Study the drawing (mm; zero at the part's minimum x, y, z) and answer. A direction names the side the tool comes from. Round coordinates to 2 decimals unless told otherwise and drop trailing zeros. Order: outer loops, then holes, each group sorted by start corner. A loop starts at its lowest first (then second) coordinate and runs counter-clockwise, first axis right, second up. Notation, with made-up numbers: (84, 76.25) - (97, 76.25) arc R27 ccw to (97, 110.25) - close; hole circle Ø1 at (-24, 48.5). An arc over 180 degrees is marked (long way). Put each result on its own line as item: value.
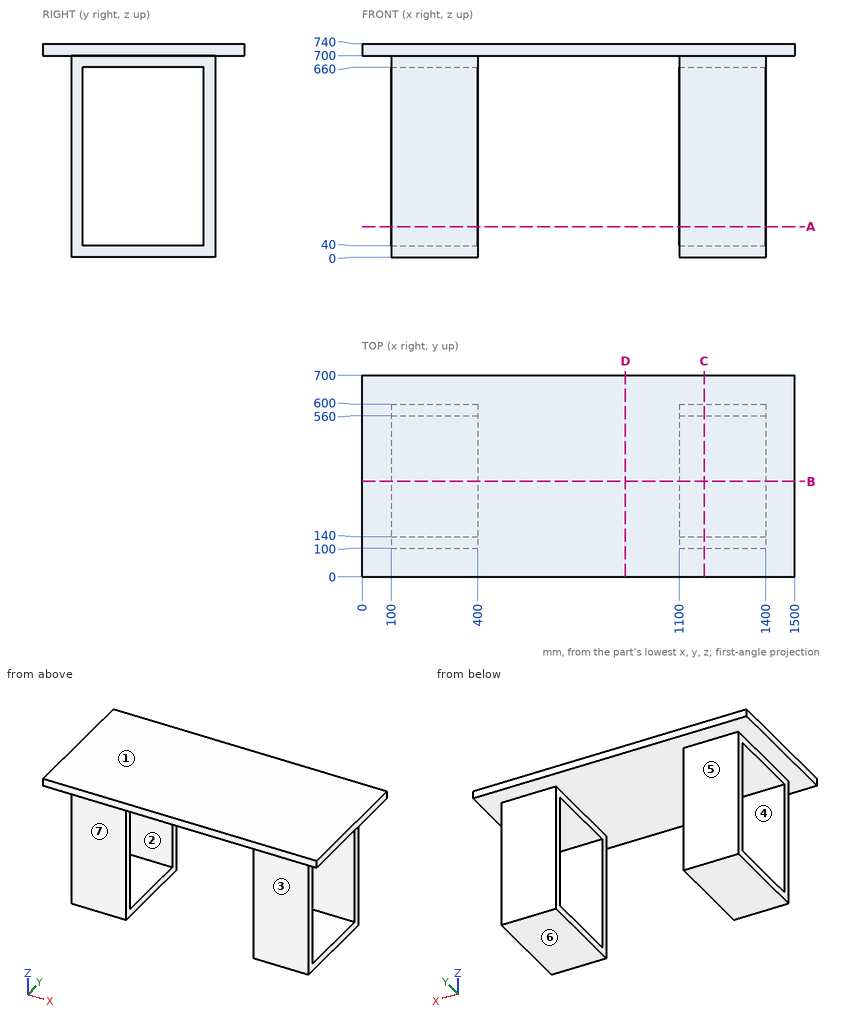
1) Straight lines are drawn through the part: L1, parallel to Z at x = 1194, y = 204; L2, parallel to Y at x = 192, z = 152.5; L3, parallel to Z at x = 1039, y = 37. For each, find the intervals that lie inside material, in ascending order. Write a range as from..to.
Findings below:
L1: z = 0..40, 660..740
L2: y = 100..140, 560..600
L3: z = 700..740
2) For a pull along Z with two mould halves and no side action, classify the marked faces 1, 2 and 3 as pulls with the +Z half, pulls with the -Z half, needs draft (parallel to the pull), parting line crosses it, or undercut.
Findings below:
face 1: pulls with the +Z half
face 2: undercut
face 3: needs draft
3) A cutting plane is placed at A-A on z = 106.5. Write down the section's boundary in (x, y), then the cut area to 3 significant figures.
Findings below:
outline: (100, 100) - (400, 100) - (400, 140) - (100, 140) - close; (100, 560) - (400, 560) - (400, 600) - (100, 600) - close; (1100, 100) - (1400, 100) - (1400, 140) - (1100, 140) - close; (1100, 560) - (1400, 560) - (1400, 600) - (1100, 600) - close
area: 48,000 mm2
4) For the marked faces 4, 5, 6 and 7, determine the directions among +Z, -Z, +X, -X, +Y, -Y from which every point of the face is accessible in a straight line to the end or side of a thin tool.
Findings below:
face 4: +X, -X
face 5: -Z, +X, -X, +Y
face 6: -Z, +X, -X, +Y, -Y
face 7: -Z, +X, -X, -Y
5) A cutting plane is placed at B-B on y = 331.5. Write down the section's boundary in (x, z).
Findings below:
outline: (0, 700) - (100, 700) - (100, 660) - (400, 660) - (400, 700) - (1100, 700) - (1100, 660) - (1400, 660) - (1400, 700) - (1500, 700) - (1500, 740) - (0, 740) - close; (100, 0) - (400, 0) - (400, 40) - (100, 40) - close; (1100, 0) - (1400, 0) - (1400, 40) - (1100, 40) - close
6) Given pin 1 Ø10 at (x, y) = (1270.5, 430) entering from -Z; pin 2 Ø1.5 at (x, z) = (355.5, 513.5) entering from -Y; pin 3 Ø6 at (x, z) = (1267, 436) entering from +Y; pin 4 Ø10 at (x, y) = (423, 172.5) entering from -Z, each flat-ended and moving along its own axis, determine where each tip first touches the part or whether it passes through.
Findings below:
pin 1: stops at z = 0
pin 2: stops at y = 100
pin 3: stops at y = 600
pin 4: stops at z = 700
7) A cutting plane is placed at C-C on x = 1186.5. Write down the section's boundary in (y, z).
Findings below:
outline: (0, 700) - (100, 700) - (100, 0) - (600, 0) - (600, 700) - (700, 700) - (700, 740) - (0, 740) - close; hole (140, 40) - (560, 40) - (560, 660) - (140, 660) - close
8) A cutting plane is placed at D-D on x = 913. Write down the section's boundary in (y, z), then the cut area to 3 significant figures.
Findings below:
outline: (0, 700) - (700, 700) - (700, 740) - (0, 740) - close
area: 28,000 mm2
